Design review of the part built by this model. Coordinates are the model's own, in mm. Coordinates: 2 decimals unless noted, no trailing zeros. Loops run counter-clockwise (first coordinate to the right, second up) from the corner with the lowest first, then second, coordinate; pieces in that order, holes last. Notation, with made-up numbers: (41, -35.5) - (53, -35.5) arc R29 cw to (53, -14.5) - close; hole circle Ø1 at (-28, -32.75). An arc over 180 degrees is marked (long way). Use one line per item in the form item = value. Start each with the question number.
(1) Add section C-C (y = 25). State the section outline as (x, z) points, plus the area to 3 significant figures.
(2) Add section A-A (x = 0). State the section outline as (y, z) points, plus the area to 3 significant figures.
(3) Clearance check with flat-ended pins moving along their axes: pin 1 Ø2 at (x, z) = (19.5, 5) entering from -Y; pin 2 Ø4 at (x, y) = (-30, 25) entering from -Z; pin 3 Ø1.5 at (y, z) = (-43.5, 4.5) entering from +X. State where each tip first meets the part, or that it passes through.
(4) Add section B-B (y = -40). State the section outline as (x, z) points, plus the area to 4 significant figures.
(5) For L1, parallel to Z at x = -62, y = -40; L2, parallel to Y at x = 65.5, z = 5.25; L3, parallel to Y at x = -35.5, z = 5.75, list the stretches that pass through material, from the lowest coordinate up.
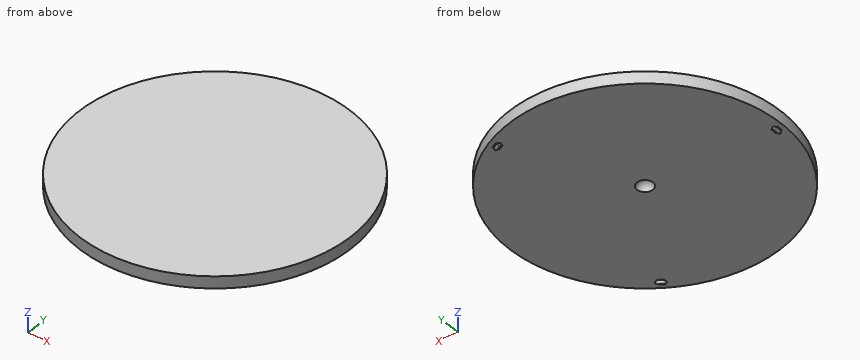
```python
from build123d import *

# Parameters (mm, degrees)
SKETCH1_R                = 85
BOSS_EXTRUDE1_DEPTH      = 7.5
CUT_EXTRUDE1_DEPTH       = 2
SKETCH4_R                = 1
BOSS_EXTRUDE2_DEPTH      = 2
REVOLVE1_ANGLE           = 90
CIRPATTERN1_COUNT        = 3
CIRPATTERN1_COPY_1_ANGLE = 90
CIRPATTERN1_COPY_2_ANGLE = 90


with BuildPart() as part:
    # Sketch1 → Boss-Extrude1 (new body)
    with BuildSketch(Plane.XY):
        Circle(SKETCH1_R)
    extrude(amount=BOSS_EXTRUDE1_DEPTH)

    # Sketch3 → Cut-Extrude1 (cut, symmetric)
    with BuildSketch(Plane(origin=(0, 0, -92.825007953), x_dir=(0, 0, -1), z_dir=(-0.837169104, -0.546944139, 0))):
        with BuildLine():
            Line((-92.825007953, 82), (-92.825007953, 78))
            ThreePointArc((-92.825007953, 78), (-94.825007953, 80), (-92.825007953, 82))
        make_face()
    cut_extrude1 = extrude(amount=CUT_EXTRUDE1_DEPTH, both=True, mode=Mode.SUBTRACT)

    # Sketch4 → Boss-Extrude2 (add, symmetric)
    with BuildSketch(Plane(origin=(0, 0, -92.825007953), x_dir=(0, 0, -1), z_dir=(-0.837169104, -0.546944139, 0))):
        with Locations((-92.825007953, 80)):
            Circle(SKETCH4_R)
    boss_extrude2 = extrude(amount=BOSS_EXTRUDE2_DEPTH, both=True)

    # Sketch5 → Revolve1 (revolve)
    with BuildSketch(Plane(origin=(-1.674338209, -1.093888277, 0), x_dir=(0, 0, -1), z_dir=(-0.837169104, -0.546944139, 0))):
        with BuildLine():
            Line((0, 81), (0, 79))
            ThreePointArc((0, 79), (1, 80), (0, 81))
        make_face()
    revolve1 = revolve(axis=Axis((42.628137018, -68.904585728, 0), (-0.546944139, 0.837169104, 0)), revolution_arc=REVOLVE1_ANGLE)

    # Mirror1: Revolve1 across plane
    add(revolve1.mirror(Plane(origin=(0, 0, 0), x_dir=(0, 0, 1), z_dir=(0.837169104, 0.546944139, 0))))

    # CirPattern1: Cut-Extrude1, Boss-Extrude2, Revolve1 ×3 about axis
    cirpattern1_axis = Axis((0, 0, 0), (0, 0, 1))
    for i in range(1, CIRPATTERN1_COUNT):
        add(cut_extrude1.rotate(cirpattern1_axis, i * 360 / CIRPATTERN1_COUNT), mode=Mode.SUBTRACT)
        add(boss_extrude2.rotate(cirpattern1_axis, i * 360 / CIRPATTERN1_COUNT))
        add(revolve1.rotate(cirpattern1_axis, i * 360 / CIRPATTERN1_COUNT))

    # CirPattern1 copy 1 sketch → CirPattern1 copy 1 (revolve)
    with BuildSketch(Plane(origin=(-1.784504141, 0.903075285, 0), x_dir=(0, 0, -1), z_dir=(-0.892252071, 0.451537642, 0))):
        with BuildLine():
            Line((0, -81), (0, -79))
            ThreePointArc((0, -79), (1, -80), (0, -81))
        make_face()
    revolve(axis=Axis((34.790044886, 73.175493007, 0), (0.451537642, 0.892252071, 0)), revolution_arc=CIRPATTERN1_COPY_1_ANGLE)

    # CirPattern1 copy 2 sketch → CirPattern1 copy 2 (revolve)
    with BuildSketch(Plane(origin=(0.110165933, -1.996963562, 0), x_dir=(0, 0, -1), z_dir=(0.055082966, -0.998481781, 0))):
        with BuildLine():
            Line((0, -81), (0, -79))
            ThreePointArc((0, -79), (1, -80), (0, -81))
        make_face()
    revolve(axis=Axis((-80.766858322, -6.458683833, 0), (-0.998481781, -0.055082966, 0)), revolution_arc=CIRPATTERN1_COPY_2_ANGLE)

    # Sketch6 → Cut-Revolve1 (revolve, cut)
    with BuildSketch(Plane(origin=(0, 0, 0), x_dir=(0, 0, -1), z_dir=(1, 0, 0))):
        with BuildLine():
            Line((5, 0), (-5, 0))
            ThreePointArc((-5, 0), (0, 5), (5, 0))
        make_face()
    revolve(axis=Axis((0, 0, -5), (0, 0, 1)), mode=Mode.SUBTRACT)


solid = part.part
```
Computed values:
q1.outline = (-81.24, 0) - (81.24, 0) - (81.24, 7.5) - (-81.24, 7.5) - close
q1.area = 1,220 mm^2
q2.outline = (-85, 0) - (-5, 0) arc R5 cw to (5, 0) - (85, 0) - (85, 7.5) - (-85, 7.5) - close
q2.area = 1,240 mm^2
q3.pin_1 = -82.96
q3.pin_2 = 0
q3.pin_3 = 73.47
q4.outline = (-75, 0) - (75, 0) - (75, 7.5) - (-75, 7.5) - close
q4.area = 1,125 mm^2
q5.L1 = 0 to 7.5
q5.L2 = -54.17 to 54.17
q5.L3 = -77.23 to 77.23
